For this review, take the finished solid that the model builds, in its own axes (mm). A direction names the side the tool comes from. Coordinates: 2 decimals unless noted, no trailing zeros. Order: outer loops, then holes, each group sorted by start corner. A loop starts at its lowest first (then second) coordinate and runs counter-clockwise, first axis right, second up.
from build123d import *

# Parameters (mm, degrees)
SKETCH1_R           = 50
BOSS_EXTRUDE1_DEPTH = 25
CHAMFER1_SIZE       = 10
SKETCH7_R           = 50
SKETCH8_R           = 35
SKETCH9_R           = 15
BOSS_EXTRUDE5_DEPTH = 10


with BuildPart() as part:
    # Sketch1 → Boss-Extrude1 (new body)
    with BuildSketch(Plane(origin=(0, 0, 0), x_dir=(1, 0, 0), z_dir=(0, 1, 0))):
        Circle(SKETCH1_R)
    extrude(amount=BOSS_EXTRUDE1_DEPTH)

    # Chamfer1
    chamfer1_edges = [part.edges().sort_by_distance(p)[0] for p in [
        (-50, 25, 0),
    ]]
    chamfer(chamfer1_edges, length=CHAMFER1_SIZE)

    # Sketch7 → Loft1 section 0
    with BuildSketch(Plane(origin=(0, 25, 0), x_dir=(1, 0, 0), z_dir=(0, 1, 0))):
        Circle(SKETCH7_R)
    # Sketch8 → Loft1 section 1
    with BuildSketch(Plane(origin=(0, 32, 0), x_dir=(1, 0, 0), z_dir=(0, 1, 0))):
        Circle(SKETCH8_R)
    loft()

    # Sketch9 → Boss-Extrude5 (add)
    with BuildSketch(Plane(origin=(0, 32, 0), x_dir=(1, 0, 0), z_dir=(0, 1, 0))):
        Circle(SKETCH9_R)
    extrude(amount=BOSS_EXTRUDE5_DEPTH)


solid = part.part
1. To check wall thickness, follow L1, parallel to Y at x = -1, z = 30; L2, parallel to X at y = 11.5, z = 0.5; L3, parallel to X at y = 40, z = 0.5. State the ranges of each line that lie inside material, in increasing order.
Answer below:
L1: y = 0 to 32
L2: x = -50 to 50
L3: x = -14.99 to 14.99
2. Clearance check with flat-ended pins moving along their axes: pin 1 Ø2 at (x, y) = (-34.5, 6) entering from -Z; pin 2 Ø1.5 at (x, y) = (21, 17) entering from -Z; pin 3 Ø6 at (x, z) = (29.5, -2.5) entering from -Y; pin 4 Ø2 at (x, y) = (-12, 37.5) entering from -Z. State where each tip first meets the part, or that it passes through.
Answer below:
pin 1: stops at z = -37.12
pin 2: stops at z = -44.07
pin 3: stops at y = 0
pin 4: stops at z = -10.2
3. Take a section at A-A, the plane x = 0. Give the boundary of the cut face in (y, z), plus the area to 4 significant figures.
Answer below:
outline: (0, -50) - (15, -50) - (25, -40) - (25, -50) - (32, -35) - (32, -15) - (42, -15) - (42, 15) - (32, 15) - (32, 35) - (25, 50) - (25, 40) - (15, 50) - (0, 50) - close
area: 3,295 mm2
4. Take a section at C-C, the plane y = 21. Give the boundary of the cut face in (x, z), plus the area to 3 significant figures.
Answer below:
outline: circle Ø88 at (0, 0)
area: 6,080 mm2
5. Take a section at B-B, the plane y = 12. Give the boundary of the cut face in (x, z).
Answer below:
outline: circle Ø100 at (0, 0)
6. Machinability: for faces 1 (the face through (-14.985, 36.93, -0.66)), 2 (the face through (47.69, 7.4, -15.02)), 3 (the face through (-32.128, 24.514, 24.635)), which of the approach directions +Z, -Z, +X, -X, +Y, -Y give a long, thin tool a straight path to every point of the face, cutting with its end or side? Answer none if there is none.
Answer below:
face 1: +Y
face 2: +Y, -Y
face 3: none
